from build123d import *

# Parameters (mm, degrees)
EXTRUDE1_DEPTH            = 80
M8_7_8_7_DIAMETER_HOLE1_D = 8.7
HOLE1_D                   = 5
HOLE1_CBORE_D             = 8
HOLE1_CBORE_DEPTH         = 3
HOLE2_D                   = 5
HOLE2_DEPTH               = 7
HOLE2_CBORE_D             = 8
HOLE2_CBORE_DEPTH         = 3


with BuildPart() as part:
    # Sketch2 → Extrude1 (new body)
    with BuildSketch(Plane.XY):
        with BuildLine():
            Line((153.422248213, 153.636884267), (59.422248213, 153.636884267))
            Line((59.422248213, 153.636884267), (59.422248213, 144.111884267))
            Line((59.422248213, 144.111884267), (76.872248213, 144.111884267))
            ThreePointArc((76.872248213, 144.111884267), (78.993568556, 143.233204611), (79.872248213, 141.111884267))
            Line((79.872248213, 141.111884267), (79.872248213, 113.299884267))
            Line((79.872248213, 113.299884267), (86.222248213, 113.299884267))
            Line((86.222248213, 113.299884267), (86.222248213, 138.349884267))
            Line((86.222248213, 138.349884267), (86.222248213, 143.499884267))
            ThreePointArc((86.222248213, 143.499884267), (87.100927869, 145.621204611), (89.222248213, 146.499884267))
            Line((89.222248213, 146.499884267), (94.372248213, 146.499884267))
            Line((94.372248213, 146.499884267), (118.472248213, 146.499884267))
            Line((118.472248213, 146.499884267), (123.622248213, 146.499884267))
            ThreePointArc((123.622248213, 146.499884267), (125.743568556, 145.621204611), (126.622248213, 143.499884267))
            Line((126.622248213, 143.499884267), (126.622248213, 138.349884267))
            Line((126.622248213, 138.349884267), (126.622248213, 113.299884267))
            Line((126.622248213, 113.299884267), (132.972248213, 113.299884267))
            Line((132.972248213, 113.299884267), (132.972248213, 141.111884267))
            ThreePointArc((132.972248213, 141.111884267), (133.850927869, 143.233204611), (135.972248213, 144.111884267))
            Line((135.972248213, 144.111884267), (153.422248213, 144.111884267))
            Line((153.422248213, 144.111884267), (153.422248213, 153.636884267))
        make_face()
    extrude(amount=EXTRUDE1_DEPTH)

    # M8.7 (8.7) Diameter Hole1 (through all)
    with Locations(Plane(origin=(68.922248213, 153.636884267, 65), x_dir=(1, 0, 0), z_dir=(0, 1, 0))):
        with Locations((0, 0), (0, 25), (0, 50), (75, 50), (75, 25), (75, 0)):
            Hole(M8_7_8_7_DIAMETER_HOLE1_D / 2)

    # Hole1 (through all)
    with Locations(Plane(origin=(106.422248213, 153.636884267, 65), x_dir=(1, 0, 0), z_dir=(0, 1, 0))):
        with Locations((0, 0), (0, 25), (0, 50)):
            CounterBoreHole(HOLE1_D / 2, HOLE1_CBORE_D / 2, HOLE1_CBORE_DEPTH)

    # Hole2
    with Locations(Plane(origin=(132.972248213, 126.296884267, 65), x_dir=(0, 0, 1), z_dir=(1, 0, 0))):
        with Locations((0, 0), (-25, 0), (-50, 0)):
            hole2 = CounterBoreHole(HOLE2_D / 2, HOLE2_CBORE_D / 2, HOLE2_CBORE_DEPTH, depth=HOLE2_DEPTH)

    # Mirror1: Hole2 across plane
    add(hole2.mirror(Plane.ZY.offset(-106.422248213)), mode=Mode.SUBTRACT)


solid = part.part
Verification items for the finished model (mm, model axes). A direction names the side the tool comes from. Give positions to 0.01 mm unless a question says otherwise; leave off trailing zeros. Loops run counter-clockwise (first coordinate to the right, second up) from the corner with the lowest first, then second, coordinate; pieces in that order, holes last.
1. Tool access check on faces 1 (the cylindrical face through (81.351, 122.924, 67.15)), 2 (the flat face through (132.972, 133, 39)), 3 (the flat face through (64, 144.112, 39)), 4 (the flat face through (106, 150.637, 43)), 5 (the flat face through (102, 146.5, 39)). Record the directions out of +Z, -Z, +X, -X, +Y, -Y that give a thin tool (end or side, any length) a straight path to the whole face; none if there is none.
Derived:
face 1: -X
face 2: +Z, -Z, +X, -Y
face 3: +Z, -Z, -X, -Y
face 4: +Y
face 5: +Z, -Z, -Y
2. Go/stop test with flat-tipped pins: P1, Ø4, axis at y = 125.5, z = 39, coming from the -X side; P2, Ø8, axis at y = 117.5, z = 14, coming from the +X side; P3, Ø4, axis at y = 135.5, z = 19.5, coming from the -X side; P4, Ø4, axis at y = 126.3, z = 15, coming from the +X side. Record where each tip stops, or that it passes through.
Derived:
P1: stops at x = 82.87
P2: stops at x = 132.97
P3: stops at x = 79.87
P4: passes through
3. Cross-section at A-A on y = 120.5. Record the cut outline in (x, z).
Derived:
outline: (79.87, 0) - (86.22, 0) - (86.22, 80) - (79.87, 80) - close; (126.62, 0) - (132.97, 0) - (132.97, 80) - (126.62, 80) - close
4. Release check for a two-part mould opening along Z. For faces 6 (the flat face through (83, 113.3, 39)), 7 (the flat face through (129.972, 124, 42)) record: +Z half, -Z half, draft (parallel to the pull), parting line (faces both ways), or undercut.
Derived:
face 6: draft
face 7: undercut
5. Material ranges on probe 1 along X at (y, z) = (150, 65); probe 2 along X at (y, z) = (119.5, 41.5); probe 3 along X at (y, z) = (129, 40), recorded low to high.
Derived:
probe 1: x = 59.42 to 64.57, 73.27 to 103.92, 108.92 to 139.57, 148.27 to 153.42
probe 2: x = 79.87 to 86.22, 126.62 to 132.97
probe 3: x = 82.87 to 86.22, 126.62 to 129.97
6. Cross-section at D-D on x = 120. Record the cut outline in (y, z), and give its area (3 significant figures).
Derived:
outline: (146.5, 0) - (153.64, 0) - (153.64, 80) - (146.5, 80) - close
area: 571 mm2
7. Cross-section at C-C on x = 84. Record the cut outline in (y, z).
Derived:
outline: (113.3, 0) - (153.64, 0) - (153.64, 80) - (113.3, 80) - close; hole circle Ø5 at (126.3, 15); hole circle Ø5 at (126.3, 40); hole circle Ø5 at (126.3, 65)
8. Cross-section at B-B on z = 34.5. Record the cut outline in (x, y), and give its area (3 significant figures).
Derived:
outline: (59.42, 144.11) - (76.87, 144.11) arc R3 cw to (79.87, 141.11) - (79.87, 113.3) - (86.22, 113.3) - (86.22, 143.5) arc R3 cw to (89.22, 146.5) - (123.62, 146.5) arc R3 cw to (126.62, 143.5) - (126.62, 113.3) - (132.97, 113.3) - (132.97, 141.11) arc R3 cw to (135.97, 144.11) - (153.42, 144.11) - (153.42, 153.64) - (59.42, 153.64) - close
area: 1,200 mm2
